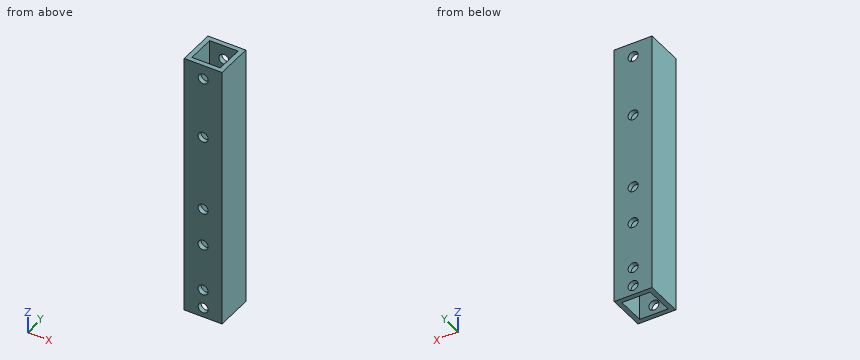
Autodesk Inventor part; units mm, degrees
ref_plane "YZ Plane" through (0, 0, 0) normal (1, 0, 0) x (0, 1, 0)
ref_plane "XZ Plane" through (0, 0, 0) normal (0, 1, 0) x (-1, 0, 0)
ref_plane "XY Plane" through (0, 0, 0) normal (0, 0, 1) x (1, 0, 0)
sketch "Sketch1" plane through (0, 0, 0) normal (0, 0, 1) x (1, 0, 0)
  line L0 (0, 0) -> (-25.4, 0)
  line L1 (-25.4, 0) -> (-25.4, 25.4)
  line L2 (-25.4, 25.4) -> (0, 25.4)
  line L3 (0, 25.4) -> (0, 0)
  line L4 (-3.175, 22.225) -> (-22.225, 22.225)
  line L5 (-22.225, 22.225) -> (-22.225, 3.175)
  line L6 (-22.225, 3.175) -> (-3.175, 3.175)
  line L7 (-3.175, 3.175) -> (-3.175, 22.225)
  dimension "d0" = 25.4
  dimension "d2" = 25.4
  dimension "d3" = 3.175
extrude "Extrusion1" add sketch "Sketch1" along normal blind 177.8
sketch "Sketch2" plane through (-25.4, 25.4, 0) normal (0, 1, 0) x (1, 0, 0)
  circle A0 centre (12.7, -19.05) radius 3.3782
  circle A1 centre (12.7, -6.35) radius 3.3782
extrude "Extrusion2" cut sketch "Sketch2" against normal blind 25.4
sketch "Sketch3" plane through (-25.4, 0, 0) normal (0, -1, 0) x (1, 0, 0)
  circle A0 centre (12.7, 76.2) radius 3.3782
  line L0 (336.55, 50.8) -> (-157.1625, 50.8)
  circle A1 centre (12.7, 50.8) radius 3.3782
extrude "Extrusion3" cut sketch "Sketch3" against normal blind 25.4
sketch "Sketch5" plane through (-25.4, 0, 0) normal (0, -1, 0) x (1, 0, 0)
  circle A0 centre (12.7, 127) radius 3.3782
  circle A1 centre (12.7, 168.275) radius 3.3782
extrude "Extrusion4" cut sketch "Sketch5" against normal blind 25.4
properties part number "winch mount" material "Aluminum 6061"
Could you check a few things on this model? Use its own coordinates, in mm. Give positions to 0.01 mm unless a question says otherwise; leave off trailing zeros. Write each loop counter-clockwise with the first axis right and the second up, starting at its lowest first coordinate (ties: lowest second). Pieces come first, ordered by that corner, then holes. Notation, with made-up numbers: (-20, 73.25) -> (28, 73.25) arc R31 ccw to (28, 99.25) -> close; hole circle Ø2 at (30.5, 72). An arc over 180 degrees is marked (long way). Write each question's results on one line, items separated by ' | '. Start each with the question number.
Q1. Suppose I cut it at C-C, the plane z = 127. List the corners of the cut face in (x, y) for me (3 decimals).
Q2. Suppose I cut it at A-A, the plane y = 17.25. List the corners of the cut face in (x, z) for me (3 decimals).
Q3. I need wall thicknesses on probe 1 along X at (y, z) = (10.5, 29) (3 decimals); probe 2 along Y at (x, z) = (-10.5, 70) (3 decimals). Which ranges of each line are inside material? Lowest first, please.
Q4. Suppose I cut it at B-B, the plane x = -18. List the corners of the cut face in (y, z) for me (3 decimals), and give its area (3 significant figures).
Outcome:
1) outline: (-25.4, 0) -> (-16.078, 0) -> (-16.078, 3.175) -> (-22.225, 3.175) -> (-22.225, 22.225) -> (-16.078, 22.225) -> (-16.078, 25.4) -> (-25.4, 25.4) -> close; (-9.322, 0) -> (0, 0) -> (0, 25.4) -> (-9.322, 25.4) -> (-9.322, 22.225) -> (-3.175, 22.225) -> (-3.175, 3.175) -> (-9.322, 3.175) -> close
2) outline: (-25.4, 0) -> (-22.225, 0) -> (-22.225, 177.8) -> (-25.4, 177.8) -> close; (-3.175, 0) -> (0, 0) -> (0, 177.8) -> (-3.175, 177.8) -> close
3) probe 1: -25.4 to -22.225, -3.175 to 0 | probe 2: 0 to 3.175, 22.225 to 25.4
4) outline: (0, 0) -> (3.175, 0) -> (3.175, 177.8) -> (0, 177.8) -> close; (22.225, 0) -> (25.4, 0) -> (25.4, 177.8) -> (22.225, 177.8) -> close | area: 1,130 mm2
